from build123d import *

# Parameters (mm, degrees)
SKETCH1_R           = 5.08
SKETCH1_R_2         = 1.778
BOSS_EXTRUDE1_DEPTH = 10.16
SKETCH2_W           = 7.62
SKETCH2_H           = 7.62
BOSS_EXTRUDE2_DEPTH = 6.35


with BuildPart() as part:
    # Sketch1 → Boss-Extrude1 (new body)
    with BuildSketch(Plane.XY):
        with BuildLine():
            Line((-6.35, 12.7), (-6.35, 10.998522628))
            ThreePointArc((-6.35, 10.998522628), (0, -12.7), (6.35, 10.998522628))
            Line((6.35, 10.998522628), (6.35, 12.7))
            Line((6.35, 12.7), (-6.35, 12.7))
        make_face()
        Circle(SKETCH1_R, mode=Mode.SUBTRACT)
        with Locations((0, 8.128)):
            Circle(SKETCH1_R_2, mode=Mode.SUBTRACT)
        with Locations((8.128, 0)):
            Circle(SKETCH1_R_2, mode=Mode.SUBTRACT)
        with Locations((0, -8.128)):
            Circle(SKETCH1_R_2, mode=Mode.SUBTRACT)
        with Locations((-8.128, 0)):
            Circle(SKETCH1_R_2, mode=Mode.SUBTRACT)
    extrude(amount=BOSS_EXTRUDE1_DEPTH)

    # Sketch2 → Boss-Extrude2 (add)
    with BuildSketch(Plane(origin=(0, 12.7, 0), x_dir=(1, 0, 0), z_dir=(0, 1, 0))):
        with Locations((0, -5.08)):
            Rectangle(SKETCH2_W, SKETCH2_H)
    extrude(amount=BOSS_EXTRUDE2_DEPTH)


solid = part.part
Part model, mm, in its own coordinate system. A direction names the side the tool comes from. Coordinates: 2 decimals unless noted, no trailing zeros. Write each loop counter-clockwise with the first axis right and the second up, starting at its lowest first coordinate (ties: lowest second). Pieces come first, ordered by that corner, then holes. Notation, with made-up numbers: M 86,-23.5 L 115,-23.5 A14 cw 115,-19.5 Z; hole C 34.25,-24.5 d10. An arc over 180 degrees is marked long. Return JSON: item names as keys, results as strings.
1. Saw through at D-D, the plane z = 5.5. Write the cut outline in (x, y).
Determined:
{"outline": "M -6.35,11 A12.7 ccw long 6.35,11 L 6.35,12.7 L 3.81,12.7 L 3.81,19.05 L -3.81,19.05 L -3.81,12.7 L -6.35,12.7 Z; hole C -8.13,0 d3.56; hole C 0,0 d10.16; hole C 0,-8.13 d3.56; hole C 0,8.13 d3.56; hole C 8.13,0 d3.56"}
2. 3-axis set-ups, long thin cutter, end or side, ignore diameter. For faces 4 (the face through (-6.35, 12, 5)), 5 (the face through (0, 16, 8.89)), 6 (the face through (3.81, 16, 5)): which of +Z, -Z, +X, -X, +Y, -Y reach the whole face in a straight line?
Determined:
{"face 4": "+Z, -Z, -X, +Y", "face 5": "+Z, +X, -X, +Y", "face 6": "+Z, -Z, +X, +Y"}
3. Pull direction Y, two halves, no side cores. Call faces 1 (the face through (-0.47, -12.69, 5.01)), 2 (the face through (0, 16, 1.27)), 3 (the face through (-0.661, 5.037, 5.009)): pulls with the +Y half, pulls with the -Y half, needs draft (parallel to the pull), parting line crosses it, or undercut.
Determined:
{"face 1": "parting line crosses it", "face 2": "needs draft", "face 3": "undercut"}
4. Saw through at B-B, the plane y = 0. Write the cut outline in (x, z).
Determined:
{"outline": "M -12.7,0 L -9.91,0 L -9.91,10.16 L -12.7,10.16 Z; M -6.35,0 L -5.08,0 L -5.08,10.16 L -6.35,10.16 Z; M 5.08,0 L 6.35,0 L 6.35,10.16 L 5.08,10.16 Z; M 9.91,0 L 12.7,0 L 12.7,10.16 L 9.91,10.16 Z"}
5. Saw through at C-C, the plane y = -7.5. Write the cut outline in (x, z).
Determined:
{"outline": "M -10.25,0 L -1.66,0 L -1.66,10.16 L -10.25,10.16 Z; M 1.66,0 L 10.25,0 L 10.25,10.16 L 1.66,10.16 Z"}
6. Saw through at A-A, the plane x = 0. Write the cut outline in (y, z).
Determined:
{"outline": "M -12.7,0 L -9.91,0 L -9.91,10.16 L -12.7,10.16 Z; M -6.35,0 L -5.08,0 L -5.08,10.16 L -6.35,10.16 Z; M 5.08,0 L 6.35,0 L 6.35,10.16 L 5.08,10.16 Z; M 9.91,0 L 12.7,0 L 12.7,1.27 L 19.05,1.27 L 19.05,8.89 L 12.7,8.89 L 12.7,10.16 L 9.91,10.16 Z"}
7. Flat gauge pins, fed straight in: pin 1 Ø1.9 at (y, z) = (15.5, 4) entering from +X; pin 2 Ø2 at (x, z) = (-6.5, 1) entering from +Y; pin 3 Ø3 at (y, z) = (6.5, 4.5) entering from -X. Where does each tip first touch, or does it go through?
Determined:
{"pin 1": "x = 3.81", "pin 2": "y = 12.7", "pin 3": "x = -11.67"}
8. Probe L1, parallel to Y at x = 0, z = 2.5; L2, parallel to X at y = -1.5, z = 0.75; L3, parallel to X at y = 14.5, z = 8. List the from-to ranges inside material, lowest first.
Determined:
{"L1": "-12.7 to -9.91, -6.35 to -5.08, 5.08 to 6.35, 9.91 to 19.05", "L2": "-12.61 to -9.08, -7.17 to -4.85, 4.85 to 7.17, 9.08 to 12.61", "L3": "-3.81 to 3.81"}
